Autodesk Fusion 360 part; units mm, degrees
sketch "Sketch1" plane through (0, 0, 0) normal (0, 1, 0) x (1, 0, 0)
  line L0 (0, 0) -> (7, 0)
  line L1 (7, 0) -> (7, -11.8)
  line L2 (7, -11.8) -> (0, -11.8)
  line L3 (0, -11.8) -> (0, 0)
  dimension "d1" = 7
  dimension "d2" = 11.8
extrude "Extrude1" add sketch "Sketch1" along normal blind 6.1
fillet "Fillet1" radius 3 12 edges at (7, 3.05, 11.8) (3.5, 0, 11.8) (0, 3.05, 11.8) (3.5, 6.1, 11.8) (7, 0, 5.9) (7, 3.05, 0) (3.5, 0, 0) (7, 6.1, 5.9) (0, 0, 5.9) (3.5, 6.1, 0) (0, 6.1, 5.9) (0, 3.05, 0)
Here's how the part is built. I have some questions about the finished solid (model axes, mm). Coordinates: 2 decimals unless noted, no trailing zeros. Order: outer loops, then holes, each group sorted by start corner. A loop starts at its lowest first (then second) coordinate and runs counter-clockwise, first axis right, second up. Notation, with made-up numbers: (80.25, 67.25) - (109.25, 67.25) arc R33 ccw to (109.25, 100.25) - close; hole circle Ø10 at (28.25, -31.75). An arc over 180 degrees is marked (long way). One line per question, with ' | ' between items. Start each with the question number.
1. I'm going to push flat-ended pins straight in: pin 1 Ø1 at (x, z) = (4.5, 9.5) entering from -Y; pin 2 Ø1 at (x, z) = (1, 9.5) entering from -Y; pin 3 Ø3 at (x, y) = (3, 5) entering from -Z. Where does each tip first touch, or does it pass through?
2. Please list where these lines run through material, in increasing order: line 1 along Z through (x, y) = (6.75, 3); line 2 along Y through (x, z) = (6, 3); line 3 along X through (y, z) = (2.25, 7.75). Write a range as [from, to].
3. If we section it at B-B (x = 3.5): Write out the boundary of the cut face in (y, z).
4. If we section it at A-A (z = 8): Write out the boundary of the cut face in (x, y).
Model answer:
1) pin 1: stops at y = 0.02 | pin 2: stops at y = 0.47 | pin 3: stops at z = 0.03
2) line 1: z = [1.8, 10] | line 2: y = [0.76, 5.34] | line 3: x = [0.1, 6.9]
3) outline: (0, 3) arc R3 ccw to (3, 0) - (3.1, 0) arc R3 ccw to (6.1, 3) - (6.1, 8.8) arc R3 ccw to (3.1, 11.8) - (3, 11.8) arc R3 ccw to (0, 8.8) - close
4) outline: (0, 3) arc R3 ccw to (3, 0) - (4, 0) arc R3 ccw to (7, 3) - (7, 3.1) arc R3 ccw to (4, 6.1) - (3, 6.1) arc R3 ccw to (0, 3.1) - close
